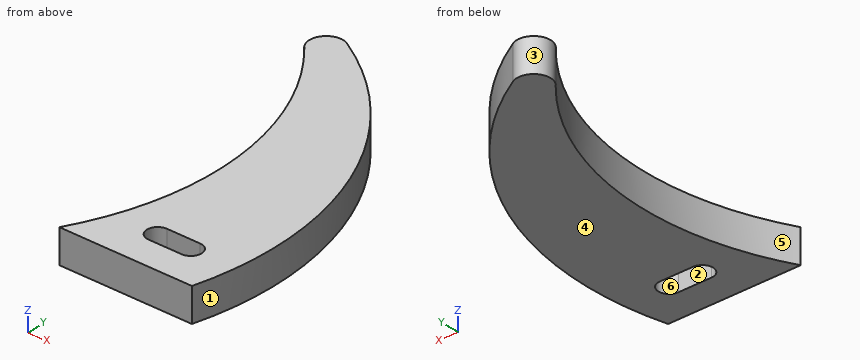
Autodesk Inventor part; units mm, degrees
ref_plane "YZ Plane" through (0, 0, 0) normal (1, 0, 0) x (0, 1, 0)
ref_plane "XZ Plane" through (0, 0, 0) normal (0, 1, 0) x (-1, 0, 0)
ref_plane "XY Plane" through (0, 0, 0) normal (0, 0, 1) x (1, 0, 0)
sketch "Sketch1" plane through (0, 0, 0) normal (0, 0, 1) x (1, 0, 0)
  arc A0 (6.3455, 7.6592) -> (3.4138, 3.6532) centre (5.1207, 5.4798) ccw
  line L0 (18.4294, -37.0751) -> (23.4294, -37.0751)
  line L1 (23.4294, -40.2751) -> (18.4294, -40.2751)
  arc A1 (18.4294, -37.0751) -> (18.4294, -40.2751) centre (18.4294, -38.6751) ccw
  arc A2 (23.4294, -40.2751) -> (23.4294, -37.0751) centre (23.4294, -38.6751) ccw
  arc A3 (29.0127, -44.8588) -> (6.3455, 7.6592) centre (-16.7656, -33.4664) ccw
  arc A4 (9.0127, -44.8588) -> (3.4138, 3.6532) centre (-28.5567, -24.6156) ccw
  line L2 (9.0127, -44.8588) -> (29.0127, -44.8588)
  point P0 (0, 0)
  dimension "d20" = 3.2
  dimension "d25" = 2.5
  dimension "d32" = 20
  dimension "d35" = 5
extrude "Extrusion1" add sketch "Sketch1" along normal blind 5
properties part number "mavac_ruka I guesss"
The model under review builds one solid part; all positions refer to its coordinate system, in mm. Face numbers are marked on the shaded views. A direction names the side the tool comes from. Give positions to 0.01 mm unless a question says otherwise; leave off trailing zeros. Order: outer loops, then holes, each group sorted by start corner. A loop starts at its lowest first (then second) coordinate and runs counter-clockwise, first axis right, second up. Notation, with made-up numbers: M -29,1 L 16,1 A26 ccw 16,36 Z; hole C -9,-6.5 d9. An arc over 180 degrees is marked long. Answer in a Markdown table with one row per item. Add a question column.
1. To check wall thickness, follow line 1 along X through (y, z) = (-39.5, 0.65); line 2 along Y through (x, z) = (18.25, 0.35); line 3 along Y through (x, z) = (20, 4.75). State the ranges of each line that lie inside material, in increasing order.
2. Mouldability with a two-part tool opening along X and no side actions: class the marked faces 1, 2, 3 and 4 as released by +X, released by -X, zero draft, split by the parting line, or undercut.
3. Machinability: for the marked faces 5 and 6, which of the approach directions +Z, -Z, +X, -X, +Y, -Y give a long, thin tool a straight path to every point of the face, cutting with its end or side? Answer none if there is none.
4. Add section D-D on x = 11.75. State the section outline as (y, z) points, plus the area to 3 significant figures.
5. For pin 1 Ø2 at (x, y) = (13.5, -33.5) entering from -Z; pin 2 Ø2.5 at (x, z) = (21, 3) entering from +Y; pin 3 Ø2 at (x, z) = (6.5, 4.5) entering from +Y; pin 4 Ø2 at (y, z) = (-16.5, 4) entering from +X, all flat-tipped, find the tip position at first contact; note any pin that passes through.
6. Add section B-B on x = 17.5. State the section outline as (y, z) points, plus the area to 3 significant figures.
7. Add section C-C on y = -3. State the section outline as (x, z) points, plus the area to 3 significant figures.
8. Add section A-A on z = 3.95. State the section outline as (x, y) points, plus the area to 3 significant figures.
The answers:
| question | item | result |
|---|---|---|
| 1 | line 1 | 11.44 to 17.06, 24.8 to 30.02 |
| 1 | line 2 | -44.86 to -40.27, -37.09 to -1.85 |
| 1 | line 3 | -44.86 to -40.28, -37.08 to -3.91 |
| 2 | face 1 | released by +X |
| 2 | face 2 | undercut |
| 2 | face 3 | split by the parting line |
| 2 | face 4 | zero draft |
| 3 | face 5 | +Z, -Z, -X |
| 3 | face 6 | +Z, -Z |
| 4 | outline | M -44.86,0 L -38.64,0 L -38.64,5 L -44.86,5 Z; M -10.59,0 L 4.11,0 L 4.11,5 L -10.59,5 Z |
| 4 | area | 105 mm2 |
| 5 | pin 1 | z = 0 |
| 5 | pin 2 | y = -3.6 |
| 5 | pin 3 | y = 7.95 |
| 5 | pin 4 | x = 27.62 |
| 6 | outline | M -44.86,0 L -39.98,0 L -39.98,5 L -44.86,5 Z; M -37.37,0 L -1.04,0 L -1.04,5 L -37.37,5 Z |
| 6 | area | 206 mm2 |
| 7 | outline | M 8.24,0 L 19.25,0 L 19.25,5 L 8.24,5 Z |
| 7 | area | 55.1 mm2 |
| 8 | outline | M 3.41,3.65 A42.68 cw 9.01,-44.86 L 29.01,-44.86 A47.17 ccw 6.35,7.66 A2.5 ccw Z; hole M 18.43,-40.28 L 23.43,-40.28 A1.6 ccw 23.43,-37.08 L 18.43,-37.08 A1.6 ccw Z |
| 8 | area | 714 mm2 |
